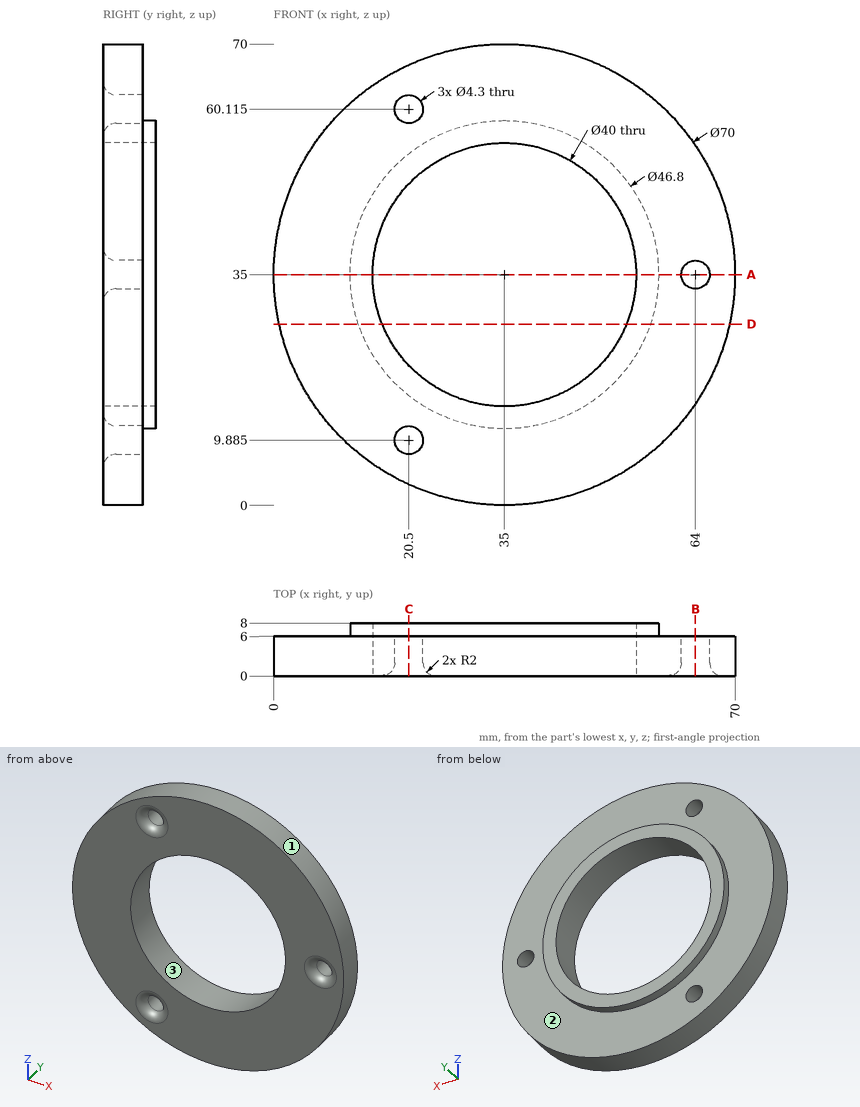
Verification items for this drawing (mm, ordinates from the low corner). Give positions to 0.01 mm unless a question says otherwise; leave off trailing zeros. Order: outer loops, then holes, each group sorted by start corner. A loop starts at its lowest first (then second) coordinate and runs counter-clockwise, first axis right, second up.
1) Cross-section at A-A (z = 35). Record the boundary of the cut face in (x, y).
Results are:
outline: (0, 0) - (15, 0) - (15, 8) - (11.6, 8) - (11.6, 6) - (0, 6) - close; (55, 0) - (59.85, 0) arc R2 ccw to (61.85, 2) - (61.85, 6) - (58.4, 6) - (58.4, 8) - (55, 8) - close; (66.15, 2) arc R2 ccw to (68.15, 0) - (70, 0) - (70, 6) - (66.15, 6) - close
2) Draft check along Z on the marked faces 1, 2 and 3. Enter one of: released by +Z, released by -Z, zero draft, split by the parting line, or undercut.
Results are:
face 1: split by the parting line
face 2: zero draft
face 3: undercut
3) Material ranges on probe 1 along X at (y, z) = (2.5, 35); probe 2 along Y at (x, z) = (49, 11); probe 3 along X at (y, z) = (6.75, 46), recorded low to high.
Results are:
probe 1: x = 0 to 15, 55 to 61.85, 66.15 to 70
probe 2: y = 0 to 6
probe 3: x = 14.35 to 18.3, 51.7 to 55.65
4) Cross-section at D-D (z = 27.5). Record the boundary of the cut face in (x, y) (1 decimal).
Results are:
outline: (0.8, 0) - (16.5, 0) - (16.5, 8) - (12.8, 8) - (12.8, 6) - (0.8, 6) - close; (53.5, 0) - (69.2, 0) - (69.2, 6) - (57.2, 6) - (57.2, 8) - (53.5, 8) - close
5) Cross-section at C-C (x = 20.5). Record the boundary of the cut face in (y, z) (1 decimal).
Results are:
outline: (0, 3.1) - (6, 3.1) - (6, 7.7) - (2, 7.7) arc R2 ccw to (0, 5.7) - close; (0, 14) arc R2 ccw to (2, 12) - (6, 12) - (6, 16.6) - (8, 16.6) - (8, 21.2) - (0, 21.2) - close; (0, 48.8) - (8, 48.8) - (8, 53.4) - (6, 53.4) - (6, 58) - (2, 58) arc R2 ccw to (0, 56) - close; (0, 64.3) arc R2 ccw to (2, 62.3) - (6, 62.3) - (6, 66.9) - (0, 66.9) - close
6) Cross-section at B-B (x = 64). Record the boundary of the cut face in (y, z), then the cut area to 3 significant figures.
Results are:
outline: (0, 15.4) - (6, 15.4) - (6, 32.85) - (2, 32.85) arc R2 ccw to (0, 30.85) - close; (0, 39.15) arc R2 ccw to (2, 37.15) - (6, 37.15) - (6, 54.6) - (0, 54.6) - close
area: 208 mm2
7) Gauge pin test, flat ends, axial feed: pin 1 (4 mm diameter, centred on x = 33, y = 7, fed in from +Z); pin 2 (7 mm diameter, centred on x = 20.5, z = 60.11, fed in from -Y); pin 3 (2 mm diameter, centred on x = 12.5, y = 3, fed in from -Z). Record the tip position at first contact, or that the pin passes through.
Results are:
pin 1: stops at z = 70
pin 2: stops at y = 0.11
pin 3: stops at z = 7.38
